Design review of the part built by this model. Coordinates are the model's own, in mm. Face numbers are marked on the shaded views. A direction names the side the tool comes from. Give positions to 0.01 mm unless a question says otherwise; leave off trailing zeros. Loops run counter-clockwise (first coordinate to the right, second up) from the corner with the lowest first, then second, coordinate; pieces in that order, holes last. Notation, with made-up numbers: (66, 34.25) - (117, 34.25) arc R34 cw to (117, 64.25) - close; hole circle Ø11 at (23, -26.5). An arc over 180 degrees is marked (long way). Write each question's results on one line, items separated by ' | '.
from build123d import *

# Parameters (mm, degrees)
HOLE_WIZARD_M3_1_D = 2.5


with BuildPart() as part:
    # 草图1 → 旋转1 (revolve)
    with BuildSketch(Plane.XY, mode=Mode.PRIVATE) as revolve_1_sk:
        Polygon((0, 1.5), (0, 2.75), (0.8, 2.75), (0.8, 2.45), (9, 2.45), (9, 0), (3.5, 0), (3.5, 1.5), align=None)
    revolve(revolve_1_sk.sketch.rotate(Axis((0, 0, 0), (1, 0, 0)), 90), axis=Axis((0, 0, 0), (1, 0, 0)))

    # M3 螺纹孔1 (through all)
    with Locations(Plane.ZY.offset(-3.5)):
        with Locations((0, 0)):
            Hole(HOLE_WIZARD_M3_1_D / 2)


solid = part.part
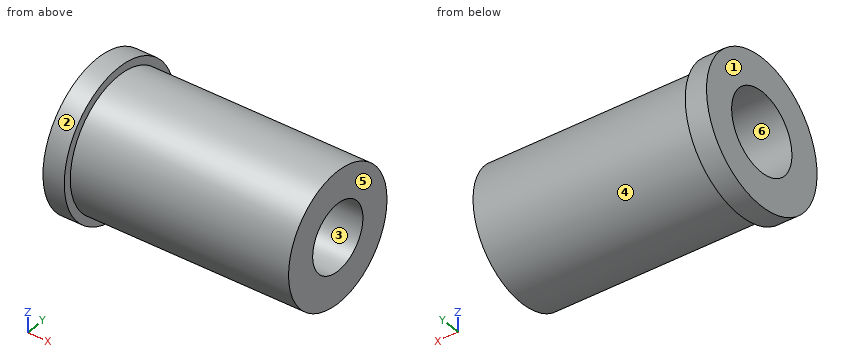
(1) Take a section at D-D on y = 1.4. Give the boundary of the cut face in (x, z), plus the area to 3 significant figures.
Answers below:
outline: (0, -2.37) - (0.8, -2.37) - (0.8, -2.01) - (9, -2.01) - (9, 2.01) - (0.8, 2.01) - (0.8, 2.37) - (0, 2.37) - (0, 0.54) - (3.5, 0.54) - (3.5, -0.54) - (0, -0.54) - close | area: 33.0 mm2
(2) Tool access review of the marked faces 4, 5 and 6: name each direction out of +Z, -Z, +X, -X, +Y, -Y from which nothing blocks a thin tool from reaching the whole face with its end or side.
Answers below:
face 4: +X | face 5: +Z, -Z, +X, +Y, -Y | face 6: -X
(3) Draft analysis for pull direction Z (two halves, no side actions). For the marked faces 1, 2 and 3, state which applies: pulls with the +Z half, pulls with the -Z half, needs draft (parallel to the pull), parting line crosses it, or undercut.
Answers below:
face 1: needs draft | face 2: parting line crosses it | face 3: undercut
(4) Take a section at C-C on x = 1.75. Give the boundary of the cut face in (y, z), plus the area to 3 significant figures.
Answers below:
outline: circle Ø4.9 at (0, 0); hole circle Ø3 at (0, 0) | area: 11.8 mm2
(5) Take a section at A-A on y = 0. Give the boundary of the cut face in (x, z).
Answers below:
outline: (0, -2.75) - (0.8, -2.75) - (0.8, -2.45) - (9, -2.45) - (9, -1.25) - (3.5, -1.25) - (3.5, -1.5) - (0, -1.5) - close; (0, 1.5) - (3.5, 1.5) - (3.5, 1.25) - (9, 1.25) - (9, 2.45) - (0.8, 2.45) - (0.8, 2.75) - (0, 2.75) - close
(6) Wall thickness on line 1 along Y through (x, z) = (1.7, 0); line 2 along X through (y, z) = (2.3, 1.25); line 3 along X through (y, z) = (-1, -0.85): over which ranges is each line inside the solid? List them lowest first. Write a range as from..to.
Answers below:
line 1: -2.45..-1.5, 1.5..2.45 | line 2: 0..0.8 | line 3: 3.5..9
(7) Insertion check: P1, Ø2, axis at x = 7.5, z = -1, coming from the -Y side; P2, Ø3, axis at x = 7.5, y = -2, coming from the -Z side. Each pin has a flat end and moves straight along its axis. Give the tip position at first contact, or say it passes through.
Answers below:
P1: y = -2.45 | P2: z = -2.4
